```python
from build123d import *

# Parameters (mm, degrees)
F1_DEPTH = 1.5
F2_R     = 6
F3_R     = 20


with BuildPart() as f1:
    # F0 (on Top) → F1 (new body)
    with BuildSketch(Plane.XY):
        Polygon((16.235917, 84.275943), (-15.764083, 84.275943), (-15.764083, 61.275943), (-9.764083, 24.275943), (-9.764083, 9.275943), (-15.764083, -27.724057), (-15.764083, -50.724057), (16.235917, -50.724057), (16.235917, -27.724057), (10.235917, 9.275943), (10.235917, 24.275943), (16.235917, 61.275943), align=None)
        with BuildLine():
            ThreePointArc((-5.764083, -43.724057), (-5.471189, -43.01695), (-4.764083, -42.724057))
            Line((-4.764083, -42.724057), (5.235917, -42.724057))
            ThreePointArc((5.235917, -42.724057), (5.943024, -43.01695), (6.235917, -43.724057))
            Line((6.235917, -43.724057), (6.235917, -44.224057))
            ThreePointArc((6.235917, -44.224057), (5.943024, -44.931164), (5.235917, -45.224057))
            Line((5.235917, -45.224057), (-4.764083, -45.224057))
            ThreePointArc((-4.764083, -45.224057), (-5.471189, -44.931164), (-5.764083, -44.224057))
            Line((-5.764083, -44.224057), (-5.764083, -43.724057))
        make_face(mode=Mode.SUBTRACT)
        with BuildLine():
            Line((5.735917, 0.775943), (-4.764083, 0.775943))
            ThreePointArc((-4.764083, 0.775943), (-5.471189, 0.48305), (-5.764083, -0.224057))
            Line((-5.764083, -0.224057), (-5.764083, -8.224057))
            ThreePointArc((-5.764083, -8.224057), (-5.471189, -8.931164), (-4.764083, -9.224057))
            Line((-4.764083, -9.224057), (5.735917, -9.224057))
            ThreePointArc((5.735917, -9.224057), (6.089471, -9.370504), (6.235917, -9.724057))
            Line((6.235917, -9.724057), (6.235917, -10.224057))
            ThreePointArc((6.235917, -10.224057), (6.089471, -10.57761), (5.735917, -10.724057))
            Line((5.735917, -10.724057), (-6.264083, -10.724057))
            ThreePointArc((-6.264083, -10.724057), (-6.971189, -10.431164), (-7.264083, -9.724057))
            Line((-7.264083, -9.724057), (-7.264083, 1.275943))
            ThreePointArc((-7.264083, 1.275943), (-6.971189, 1.98305), (-6.264083, 2.275943))
            Line((-6.264083, 2.275943), (5.735917, 2.275943))
            ThreePointArc((5.735917, 2.275943), (6.089471, 2.129496), (6.235917, 1.775943))
            Line((6.235917, 1.775943), (6.235917, 1.275943))
            ThreePointArc((6.235917, 1.275943), (6.089471, 0.92239), (5.735917, 0.775943))
        make_face(mode=Mode.SUBTRACT)
        with BuildLine():
            Line((5.735917, 42.775943), (-4.764083, 42.775943))
            ThreePointArc((-4.764083, 42.775943), (-5.471189, 42.48305), (-5.764083, 41.775943))
            Line((-5.764083, 41.775943), (-5.764083, 33.775943))
            ThreePointArc((-5.764083, 33.775943), (-5.471189, 33.068836), (-4.764083, 32.775943))
            Line((-4.764083, 32.775943), (5.735917, 32.775943))
            ThreePointArc((5.735917, 32.775943), (6.089471, 32.629496), (6.235917, 32.275943))
            Line((6.235917, 32.275943), (6.235917, 31.775943))
            ThreePointArc((6.235917, 31.775943), (6.089471, 31.42239), (5.735917, 31.275943))
            Line((5.735917, 31.275943), (-6.264083, 31.275943))
            ThreePointArc((-6.264083, 31.275943), (-6.971189, 31.568836), (-7.264083, 32.275943))
            Line((-7.264083, 32.275943), (-7.264083, 43.275943))
            ThreePointArc((-7.264083, 43.275943), (-6.971189, 43.98305), (-6.264083, 44.275943))
            Line((-6.264083, 44.275943), (5.735917, 44.275943))
            ThreePointArc((5.735917, 44.275943), (6.089471, 44.129496), (6.235917, 43.775943))
            Line((6.235917, 43.775943), (6.235917, 43.275943))
            ThreePointArc((6.235917, 43.275943), (6.089471, 42.92239), (5.735917, 42.775943))
        make_face(mode=Mode.SUBTRACT)
        with BuildLine():
            Line((5.235917, 76.275943), (-4.764083, 76.275943))
            ThreePointArc((-4.764083, 76.275943), (-5.471189, 76.568836), (-5.764083, 77.275943))
            Line((-5.764083, 77.275943), (-5.764083, 77.775943))
            ThreePointArc((-5.764083, 77.775943), (-5.471189, 78.48305), (-4.764083, 78.775943))
            Line((-4.764083, 78.775943), (5.235917, 78.775943))
            ThreePointArc((5.235917, 78.775943), (5.943024, 78.48305), (6.235917, 77.775943))
            Line((6.235917, 77.775943), (6.235917, 77.275943))
            ThreePointArc((6.235917, 77.275943), (5.943024, 76.568836), (5.235917, 76.275943))
        make_face(mode=Mode.SUBTRACT)
    extrude(amount=F1_DEPTH)

    # F2
    f2_edges = [f1.edges().sort_by_distance(p)[0] for p in [
        (16.235917, 84.275943, 0.75),
        (-15.764083, 84.275943, 0.75),
        (-15.764083, -50.724057, 0.75),
        (16.235917, -50.724057, 0.75),
    ]]
    fillet(f2_edges, radius=F2_R)

    # F3
    f3_edges = [f1.edges().sort_by_distance(p)[0] for p in [
        (16.235917, 61.275943, 0.75),
        (-15.764083, 61.275943, 0.75),
        (16.235917, -27.724057, 0.75),
        (-15.764083, -27.724057, 0.75),
        (-9.764083, 9.275943, 0.75),
        (10.235917, 9.275943, 0.75),
        (10.235917, 24.275943, 0.75),
        (-9.764083, 24.275943, 0.75),
    ]]
    fillet(f3_edges, radius=F3_R)


solid = f1.part
```
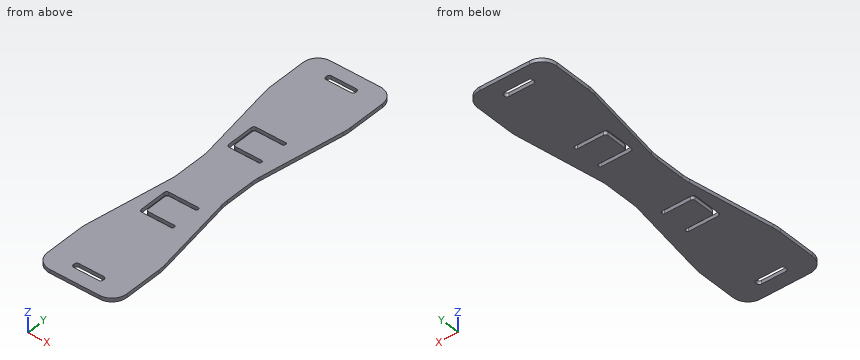
Geometry: final body of the model. Coordinates: model frame, mm. Give positions to 0.01 mm unless a question says otherwise; leave off trailing zeros. Write each loop counter-clockwise with the first axis right and the second up, starting at its lowest first coordinate (ties: lowest second). Pieces come first, ordered by that corner, then holes.
1. Section query C-C, the plane y = 36.5. Return loops of the section in (x, z).
2. Pin query (flat end, axial travel): P1, Ø0.8, axis at y = 15, z = 1, coming from the +X side; P2, Ø1, axis at x = 9.5, y = 44, coming from the -Z side. Return the tip coordinate at first contact, or that it passes through.
3. Section query D-D, the plane z = 1.2. Count the separate pieces of the cut face and the enclosed holes in it, then the cut area to 3 significant figures.
4. Section query A-A, the plane x = 3.5. Return loops of the section in (y, z), then the cut area to 3 significant figures.
5. Line query: probe 1 along X at (y, z) = (-7, 0.1); probe 2 along X at (y, z) = (34.5, 0.7); probe 3 along X at (y, z) = (53, 0.4). Output: solid intervals per line, ascending.
6. Section query B-B, the plane x = -12.5. Return loops of the section in (y, z).
Computed:
1. outline: (-11.75, 0) - (-7.26, 0) - (-7.26, 1.5) - (-11.75, 1.5) - close; (-5.76, 0) - (12.22, 0) - (12.22, 1.5) - (-5.76, 1.5) - close
2. P1: stops at x = 10.24
2. P2: stops at z = 0
3. separate pieces: 1
3. enclosed holes: 4
3. area: 3,500 mm2
4. outline: (-50.72, 0) - (-45.22, 0) - (-45.22, 1.5) - (-50.72, 1.5) - close; (-42.72, 0) - (-10.72, 0) - (-10.72, 1.5) - (-42.72, 1.5) - close; (-9.22, 0) - (0.78, 0) - (0.78, 1.5) - (-9.22, 1.5) - close; (2.28, 0) - (31.28, 0) - (31.28, 1.5) - (2.28, 1.5) - close; (32.78, 0) - (42.78, 0) - (42.78, 1.5) - (32.78, 1.5) - close; (44.28, 0) - (76.28, 0) - (76.28, 1.5) - (44.28, 1.5) - close; (78.78, 0) - (84.28, 0) - (84.28, 1.5) - (78.78, 1.5) - close
4. area: 186 mm2
5. probe 1: x = -12.4 to -7.26, -5.76 to 12.88
5. probe 2: x = -11.42 to -7.26, -5.76 to 11.89
5. probe 3: x = -14.42 to 14.89
6. outline: (-50.06, 0) - (-7.6, 0) - (-7.6, 1.5) - (-50.06, 1.5) - close; (41.15, 0) - (83.62, 0) - (83.62, 1.5) - (41.15, 1.5) - close
